from build123d import *

# Parameters (mm, degrees)
PAD_DEPTH    = 3
SKETCH001_R  = 3.1
POCKET_DEPTH = 2
SKETCH004_R  = 3.1
SKETCH005_R  = 3.5
SKETCH002_R  = 5.55
SKETCH003_R  = 7


with BuildPart() as tasche_magnet:
    # Sketch → Pad (new body)
    with BuildSketch(Plane.YZ):
        with BuildLine():
            ThreePointArc((5.499797, -0.744805), (1e-06, 5.55), (-5.499797, -0.744803))
            Line((-5.499797, -0.744803), (-3.963815, -12.086812))
            ThreePointArc((-3.963815, -12.086812), (-1e-06, -15.55), (3.963815, -12.086815))
            Line((5.499797, -0.744805), (3.963815, -12.086815))
        make_face()
    extrude(amount=PAD_DEPTH)

    # Sketch001 → Pocket (cut)
    with BuildSketch(Plane.YZ.offset(3)):
        Circle(SKETCH001_R)
    extrude(amount=-POCKET_DEPTH, mode=Mode.SUBTRACT)


with BuildPart() as loft001:
    # Sketch004 → Loft001 section 0
    with BuildSketch(Plane.YZ.offset(3)):
        Circle(SKETCH004_R)
    # Sketch005 → Loft001 section 1
    with BuildSketch(Plane.YZ.offset(5)):
        Circle(SKETCH005_R)
    loft()


with BuildPart() as fusion:
    # Sketch002 → Loft section 0
    with BuildSketch(Plane.YZ.offset(3)):
        Circle(SKETCH002_R)
    # Sketch003 → Loft section 1
    with BuildSketch(Plane.YZ.offset(5)):
        Circle(SKETCH003_R)
    loft()

    # Cut: cut Loft001
    add(loft001.part, mode=Mode.SUBTRACT)

    # Fusion: union Tasche Magnet
    add(tasche_magnet.part)


solid = fusion.part
CAD build for the part. Positions are in the model's coordinates, mm. A direction names the side the tool comes from. Round coordinates to 2 decimals unless told otherwise and drop trailing zeros. Loops run counter-clockwise (first coordinate to the right, second up) from the corner with the lowest first, then second, coordinate; pieces in that order, holes last. Notation, with made-up numbers: M -3.75,-12.75 L 49.25,-12.75 A23 cw 49.25,11.25 Z; hole C -21,37 d8. An arc over 180 degrees is marked long. One line per question, with ' | ' between items. Start each with the question number.
Item 1: Pin check, flat tips, straight feed: pin 1 Ø5 at (y, z) = (-1, 0.5) entering from +X; pin 2 Ø3.5 at (y, z) = (0, 0) entering from +X; pin 3 Ø3 at (x, y) = (1, 2) entering from +Z. Stop position of each tip, or through.
Item 2: Cut at C-C, the plane x = 4.2. Write the cut outline in (y, z), plus the area to 3 significant figures.
Item 3: Cut at B-B, the plane x = 2.3. Write the cut outline in (y, z).
Item 4: Wall check: line 1 (Z direction, x = 2.3, y = 0); line 2 (X direction, y = 1.5, z = -11.5); line 3 (Z direction, x = 1.75, y = -1.5). Give the ranges that are in metal, low to high.
Item 5: Which spindle directions (+Z, -Z, +X, -X, +Y, -Y) get a long thin tool onto all of the face, cutting with end or side? Do faces 4 (the flat face through (0, 0, -5)), 5 (the flat face through (1.479, 4.743, -6.336)), 6 (the conical face through (3.125, 5.38, 1.694)), 7 (the flat face through (1, 0, 0)), 8 (the flat face through (1.479, -4.743, -6.336)). Say none if no direction does.
Item 6: Two-plate mould, pull along Z, no slides. Class faces 1 (the cylindrical face through (1.48, -0.08, -15.55)), 2 (the flat face through (5, 3, -3)), 3 (the cylindrical face through (2.01, 1.43, -2.75)): pulls with the +Z half, pulls with the -Z half, needs draft (parallel to the pull), parting line crosses it, or undercut.
Item 7: Cut at A-A, the plane y = 0. Write the cut outline in (x, z), plus the area to 3 significant figures.
Responses:
1) pin 1: stops at x = 5 | pin 2: stops at x = 1 | pin 3: stops at z = 5.53
2) outline: C 0,0 d12.84; hole C 0,0 d6.68 | area: 94.4 mm²
3) outline: M -5.5,-0.74 L -3.96,-12.09 A4 ccw 3.96,-12.09 L 5.5,-0.74 A5.55 ccw long Z; hole C 0,0 d6.2
4) line 1: z = -15.55 to -3.1, 3.1 to 5.55 | line 2: x = 0 to 3 | line 3: z = -15.26 to -2.71, 2.71 to 5.34
5) face 4: +Z, -Z, -X, +Y, -Y | face 5: -Z, -X, +Y | face 6: none | face 7: +X | face 8: -Z, -X, -Y
6) face 1: pulls with the -Z half | face 2: needs draft | face 3: undercut
7) outline: M 0,-15.55 L 3,-15.55 L 3,-5.55 L 5,-7 L 5,-3.5 L 3,-3.1 L 1,-3.1 L 1,3.1 L 3,3.1 L 5,3.5 L 5,7 L 3,5.55 L 0,5.55 Z | area: 62.8 mm²
